```python
from build123d import *

# Parameters (mm, degrees)
ESTRUSIONE_ESTRUSIONE1_DEPTH                         = 170
FORO_LAMATO_PER_BULLONE_M5_A_TESTA_ESAGO_D           = 4.5
FORO_LAMATO_PER_BULLONE_M5_A_TESTA_ESAGO_DEPTH       = 30
FORO_LAMATO_PER_BULLONE_M5_A_TESTA_ESAGO_CBORE_D     = 10
FORO_LAMATO_PER_BULLONE_M5_A_TESTA_ESAGO_CBORE_DEPTH = 3
FORO_LAMATO_PER_BULLONE_M5_A_TESTA_ESAGO_TIP         = 1.351936393
SCHIZZO4_W                                           = 89
SCHIZZO4_H                                           = 35
TAGLIO_ESTRUSIONE1_DEPTH                             = 170
RACCORDO1_R                                          = 6
SCHIZZO5_W                                           = 15
SCHIZZO5_H                                           = 4
ESTRUSIONE_ESTRUSIONE2_DEPTH                         = 35.5
SCHIZZO6_R                                           = 1.5
TAGLIO_ESTRUSIONE2_DEPTH                             = 32
SCHIZZO7_R                                           = 3
TAGLIO_ESTRUSIONE3_DEPTH                             = 10
SMUSSO1_SIZE                                         = 10
SMUSSO2_SIZE                                         = 2


with BuildPart() as part:
    # Schizzo1 → Estrusione-Estrusione1 (new body)
    with BuildSketch(Plane(origin=(0, 0, 0), x_dir=(0, 0, -1), z_dir=(1, 0, 0))):
        with BuildLine():
            Line((0, 0), (6, 0))
            Line((6, 0), (6, 35))
            ThreePointArc((6, 35), (6.585786438, 36.414213562), (8, 37))
            Line((8, 37), (12, 37))
            ThreePointArc((12, 37), (14.828427125, 38.171572875), (16, 41))
            Line((16, 41), (16, 65))
            Line((16, 65), (10, 65))
            Line((10, 65), (10, 45))
            ThreePointArc((10, 45), (9.414213562, 43.585786438), (8, 43))
            Line((8, 43), (5, 43))
            ThreePointArc((5, 43), (1.464466094, 41.535533906), (0, 38))
            Line((0, 38), (0, 0))
        make_face()
    extrude(amount=ESTRUSIONE_ESTRUSIONE1_DEPTH)

    # Foro lamato per Bullone M5 a testa esagonale-1
    with Locations(Plane(origin=(0, 0, -6), x_dir=(-1, 0, 0), z_dir=(0, 0, -1))):
        with Locations((-25, 19.5), (-71, 19.5)):
            CounterBoreHole(FORO_LAMATO_PER_BULLONE_M5_A_TESTA_ESAGO_D / 2, FORO_LAMATO_PER_BULLONE_M5_A_TESTA_ESAGO_CBORE_D / 2, FORO_LAMATO_PER_BULLONE_M5_A_TESTA_ESAGO_CBORE_DEPTH, depth=FORO_LAMATO_PER_BULLONE_M5_A_TESTA_ESAGO_DEPTH)
            with Locations((0, 0, -(FORO_LAMATO_PER_BULLONE_M5_A_TESTA_ESAGO_DEPTH + FORO_LAMATO_PER_BULLONE_M5_A_TESTA_ESAGO_TIP / 2))):  # 118° drill point
                Cone(0, FORO_LAMATO_PER_BULLONE_M5_A_TESTA_ESAGO_D / 2, FORO_LAMATO_PER_BULLONE_M5_A_TESTA_ESAGO_TIP, mode=Mode.SUBTRACT)

    # Schizzo4 → Taglio-Estrusione1 (cut)
    with BuildSketch(Plane(origin=(0, 0, -6), x_dir=(-1, 0, 0), z_dir=(0, 0, -1))):
        with Locations((-125.5, 17.5)):
            Rectangle(SCHIZZO4_W, SCHIZZO4_H)
    extrude(amount=-TAGLIO_ESTRUSIONE1_DEPTH, mode=Mode.SUBTRACT)

    # Raccordo1
    raccordo1_edges = [part.edges().sort_by_distance(p)[0] for p in [
        (81, 35, -3),
    ]]
    fillet(raccordo1_edges, radius=RACCORDO1_R)

    # Schizzo5 → Estrusione-Estrusione2 (add)
    with BuildSketch(Plane(origin=(0, 0, -16), x_dir=(-1, 0, 0), z_dir=(0, 0, -1))):
        with Locations((-117.5, 53)):
            Rectangle(SCHIZZO5_W, SCHIZZO5_H)
    extrude(amount=ESTRUSIONE_ESTRUSIONE2_DEPTH)

    # Schizzo6 → Taglio-Estrusione2 (cut)
    with BuildSketch(Plane(origin=(0, 55, 0), x_dir=(1, 0, 0), z_dir=(0, 1, 0))):
        with Locations(Location((117.5, 44, 0), (0, 0, 270))):
            Circle(SCHIZZO6_R)
    extrude(amount=-TAGLIO_ESTRUSIONE2_DEPTH, mode=Mode.SUBTRACT)

    # Schizzo7 → Taglio-Estrusione3 (cut)
    with BuildSketch(Plane(origin=(0, 0, -16), x_dir=(-1, 0, 0), z_dir=(0, 0, -1))):
        with Locations((-121.31, 58.175)):
            Circle(SCHIZZO7_R)
        with Locations((-113.436, 58.175)):
            Circle(SCHIZZO7_R)
    extrude(amount=-TAGLIO_ESTRUSIONE3_DEPTH, mode=Mode.SUBTRACT)

    # Smusso1
    smusso1_edges = [part.edges().sort_by_distance(p)[0] for p in [
        (117.5, 51, -16),
    ]]
    chamfer(smusso1_edges, length=SMUSSO1_SIZE - 0.0001)  # a hair under: the kernel refuses the full size

    # Smusso2
    smusso2_edges = [part.edges().sort_by_distance(p)[0] for p in [
        (110, 48.00005, -16),
        (125, 48.00005, -16),
    ]]
    chamfer(smusso2_edges, length=SMUSSO2_SIZE)


solid = part.part
```
The listing builds one solid part. Answer for the finished solid, in the listing's coordinates (mm). A direction names the side the tool comes from. Round coordinates to 2 decimals unless told otherwise and drop trailing zeros. Loops run counter-clockwise (first coordinate to the right, second up) from the corner with the lowest first, then second, coordinate; pieces in that order, holes last.
Q1. Section B-B, the plane x = 71 is taken. Determine the outline of the cut face in (y, z), then the cut area to 3 significant figures.
Q2. Find the intervals of material crossed by line 1 (Y direction, x = 121.31, z = -12.15) (3 decimals); line 2 (Z direction, x = 119.5, y = 55.5); line 3 (Z direction, x = 55.5, y = 10.5), in increasing order.
Q3. Which of the six approach directions +Z, -Z, +X, -X, +Y, -Y give full straight-line access (tool end or side, diameter ignored) to faces 1 (the face through (40, 0, -3)), 2 (the face through (70, 17, -3)), 3 (the face through (129, 35, -3)), 4 (the face through (118, 51, -39))?
Q4. For a pull along Y with two mould halves and no side action, classify faces 5 (the face through (115.817, 56.35, -13.042)), 6 (the face through (118, 55, -34)), 7 (the face through (43, 17, -6)), 8 (the face through (118, 46, -21)) as released by +Y, released by -Y, zero draft, split by the parting line, or undercut.
Q5. Given pin 1 Ø1.5 at (x, y) = (31.5, 40) entering from +Z; pin 2 Ø2 at (x, z) = (97, -9.5) entering from -Y; pin 3 Ø6.5 at (y, z) = (18, -4.5) entering from +X, each flat-ended and moving along its own axis, determine where each tip first touches the part or whether it passes through.
Q6. Section C-C, the plane z = -38.5 is taken. Determine the outline of the cut face in (x, y), then the cut area to 3 significant figures.
Q7. Section A-A, the plane y = 19.5 is taken. Determine the outline of the cut face in (x, z).
Completed:
1. outline: (0, -6) - (14.5, -6) - (14.5, -3) - (17.25, -3) - (17.25, 0) - (0, 0) - close; (21.75, -3) - (24.5, -3) - (24.5, -6) - (35, -6) arc R2 cw to (37, -8) - (37, -12) arc R4 ccw to (41, -16) - (65, -16) - (65, -10) - (45, -10) arc R2 cw to (43, -8) - (43, -5) arc R5 ccw to (38, 0) - (21.75, 0) - close
1. area: 399 mm2
2. line 1: y = 37.003 to 55.175, 61.175 to 65
2. line 2: z = -16 to -10
2. line 3: z = -6 to 0
3. face 1: +Z, -Z, +X, -X, -Y
3. face 2: -Z
3. face 3: +Z, -Z, +X, -Y
3. face 4: -Z, +X, -X, -Y
4. face 5: undercut
4. face 6: released by +Y
4. face 7: zero draft
4. face 8: released by -Y
5. pin 1: stops at z = -0.16
5. pin 2: stops at y = 37
5. pin 3: stops at x = 81
6. outline: (110, 51) - (125, 51) - (125, 55) - (110, 55) - close
6. area: 60.0 mm2
7. outline: (0, -6) - (20, -6) - (20, -3) - (22.75, -3) - (22.75, 0) - (0, 0) - close; (27.25, -3) - (30, -3) - (30, -6) - (66, -6) - (66, -3) - (68.75, -3) - (68.75, 0) - (27.25, 0) - close; (73.25, -3) - (76, -3) - (76, -6) - (81, -6) - (81, 0) - (73.25, 0) - close
